Input: part model. Units: mm. Frame: model coordinates. A direction names the side the tool comes from. Coordinates: 2 decimals unless noted, no trailing zeros. Order: outer loops, then holes, each group sorted by start corner. A loop starts at its lowest first (then second) coordinate and runs counter-clockwise, first axis right, second up.
from build123d import *

# Parameters (mm, degrees)
BASE_DEPTH                  = 2
MUR_DEPTH                   = 15
ESQUISSE3_W                 = 4.5
ESQUISSE3_H                 = 4.5
FIXATION_VIS_DEPTH          = 13
CONG_1_R                    = 2
ESQUISSE4_R                 = 2.2
INSERT_M3_DEPTH             = 6
INSERT_M3_DIRECTION_2_REACH = 29.951
PASSE_CABLE_REACH           = 38.249
ESQUISSE5_R                 = 1
ESQUISSE8_W                 = 8
ESQUISSE8_H                 = 7.5
PATES_FIXATION_DEPTH        = 2
PASSAGE_VIS_REACH           = 34.33
ESQUISSE9_R                 = 1.6
CONG_10MM_R                 = 10
CONG_2MM_R                  = 2
CONG_1_5MM_R                = 1.5


with BuildPart() as part:
    # Esquisse1 → Base (new body)
    with BuildSketch(Plane(origin=(0, 0, 0), x_dir=(1, 0, 0), z_dir=(0, 1, 0))):
        with BuildLine():
            Line((-10.5, 20), (10.5, 20))
            ThreePointArc((10.5, 20), (11.914213562, 19.414213562), (12.5, 18))
            Line((12.5, 18), (12.5, -18))
            ThreePointArc((12.5, -18), (11.914213562, -19.414213562), (10.5, -20))
            Line((10.5, -20), (-10.5, -20))
            ThreePointArc((-10.5, -20), (-11.914213562, -19.414213562), (-12.5, -18))
            Line((-12.5, -18), (-12.5, 18))
            ThreePointArc((-12.5, 18), (-11.914213562, 19.414213562), (-10.5, 20))
        make_face()
    extrude(amount=BASE_DEPTH)

    # Esquisse2 → Mur (add)
    with BuildSketch(Plane(origin=(0, 2, 0), x_dir=(1, 0, 0), z_dir=(0, 1, 0))):
        with BuildLine():
            Line((-12.5, 18), (-12.5, -18))
            ThreePointArc((-12.5, -18), (-11.914213562, -19.414213562), (-10.5, -20))
            Line((-10.5, -20), (10.5, -20))
            ThreePointArc((10.5, -20), (11.914213562, -19.414213562), (12.5, -18))
            Line((12.5, -18), (12.5, 18))
            ThreePointArc((12.5, 18), (11.914213562, 19.414213562), (10.5, 20))
            Line((10.5, 20), (-10.5, 20))
            ThreePointArc((-10.5, 20), (-11.914213562, 19.414213562), (-12.5, 18))
        make_face()
        with BuildLine():
            ThreePointArc((-10.5, 18.5), (-10.853553391, 18.353553391), (-11, 18))
            Line((-11, 18), (-11, -18))
            ThreePointArc((-11, -18), (-10.853553391, -18.353553391), (-10.5, -18.5))
            Line((-10.5, -18.5), (10.5, -18.5))
            ThreePointArc((10.5, -18.5), (10.853553391, -18.353553391), (11, -18))
            Line((11, -18), (11, 18))
            ThreePointArc((11, 18), (10.853553391, 18.353553391), (10.5, 18.5))
            Line((10.5, 18.5), (-10.5, 18.5))
        make_face(mode=Mode.SUBTRACT)
    extrude(amount=MUR_DEPTH)

    # Esquisse3 → Fixation Vis (add)
    with BuildSketch(Plane(origin=(0, 2, 0), x_dir=(1, 0, 0), z_dir=(0, 1, 0))):
        with Locations((-8.75, 16.25)):
            Rectangle(ESQUISSE3_W, ESQUISSE3_H)
        with Locations((8.75, 16.25)):
            Rectangle(ESQUISSE3_W, ESQUISSE3_H)
        with Locations((8.75, -16.25)):
            Rectangle(ESQUISSE3_W, ESQUISSE3_H)
        with Locations((-8.75, -16.25)):
            Rectangle(ESQUISSE3_W, ESQUISSE3_H)
    extrude(amount=FIXATION_VIS_DEPTH)

    # Congé1
    cong_1_edges = [part.edges().sort_by_distance(p)[0] for p in [
        (6.5, 8.5, 14),
        (-6.5, 8.5, 14),
        (-6.5, 8.5, -14),
        (6.5, 8.5, -14),
    ]]
    fillet(cong_1_edges, radius=CONG_1_R)

    # Esquisse4 → Insert M3 (cut)
    with BuildSketch(Plane(origin=(0, 15, 0), x_dir=(1, 0, 0), z_dir=(0, 1, 0))):
        with Locations(Location((-9.5, 17, 0), (0, 0, 42.98588608))):
            Circle(ESQUISSE4_R)
        with Locations(Location((9.5, 17, 0), (0, 0, 90))):
            Circle(ESQUISSE4_R)
        with Locations(Location((9.5, -17, 0), (0, 0, 47.01411392))):
            Circle(ESQUISSE4_R)
        with Locations(Location((-9.5, -17, 0), (0, 0, 90))):
            Circle(ESQUISSE4_R)
    extrude(amount=-INSERT_M3_DEPTH, mode=Mode.SUBTRACT)

    # Esquisse4 → Insert M3 direction 2 (cut, up to next)
    with BuildSketch(Plane(origin=(0, 15, 0), x_dir=(1, 0, 0), z_dir=(0, 1, 0)), mode=Mode.PRIVATE) as insert_m3_direction_2_sk1:
        with Locations(Location((-9.5, 17, 0), (0, 0, 42.98588608))):
            Circle(ESQUISSE4_R)
    insert_m3_direction_2_tool1 = extrude(insert_m3_direction_2_sk1.sketch, amount=INSERT_M3_DIRECTION_2_REACH, mode=Mode.PRIVATE) & part.part
    # Esquisse4 → Insert M3 direction 2 (cut, up to next)
    with BuildSketch(Plane(origin=(0, 15, 0), x_dir=(1, 0, 0), z_dir=(0, 1, 0)), mode=Mode.PRIVATE) as insert_m3_direction_2_sk2:
        with Locations(Location((9.5, 17, 0), (0, 0, 90))):
            Circle(ESQUISSE4_R)
    insert_m3_direction_2_tool2 = extrude(insert_m3_direction_2_sk2.sketch, amount=INSERT_M3_DIRECTION_2_REACH, mode=Mode.PRIVATE) & part.part
    # Esquisse4 → Insert M3 direction 2 (cut, up to next)
    with BuildSketch(Plane(origin=(0, 15, 0), x_dir=(1, 0, 0), z_dir=(0, 1, 0)), mode=Mode.PRIVATE) as insert_m3_direction_2_sk3:
        with Locations(Location((9.5, -17, 0), (0, 0, 47.01411392))):
            Circle(ESQUISSE4_R)
    insert_m3_direction_2_tool3 = extrude(insert_m3_direction_2_sk3.sketch, amount=INSERT_M3_DIRECTION_2_REACH, mode=Mode.PRIVATE) & part.part
    # Esquisse4 → Insert M3 direction 2 (cut, up to next)
    with BuildSketch(Plane(origin=(0, 15, 0), x_dir=(1, 0, 0), z_dir=(0, 1, 0)), mode=Mode.PRIVATE) as insert_m3_direction_2_sk4:
        with Locations(Location((-9.5, -17, 0), (0, 0, 90))):
            Circle(ESQUISSE4_R)
    insert_m3_direction_2_tool4 = extrude(insert_m3_direction_2_sk4.sketch, amount=INSERT_M3_DIRECTION_2_REACH, mode=Mode.PRIVATE) & part.part
    add(insert_m3_direction_2_tool1.solids().sort_by_distance((-9.5, 15, -17))[0], mode=Mode.SUBTRACT)
    add(insert_m3_direction_2_tool2.solids().sort_by_distance((9.5, 15, -17))[0], mode=Mode.SUBTRACT)
    add(insert_m3_direction_2_tool3.solids().sort_by_distance((9.5, 15, 17))[0], mode=Mode.SUBTRACT)
    add(insert_m3_direction_2_tool4.solids().sort_by_distance((-9.5, 15, 17))[0], mode=Mode.SUBTRACT)

    # Esquisse5 → Passe-Cable (cut, up to next)
    with BuildSketch(Plane.ZY.offset(12.5), mode=Mode.PRIVATE) as passe_cable_sk1:
        with Locations((-10, 6)):
            Circle(ESQUISSE5_R)
    passe_cable_tool1 = extrude(passe_cable_sk1.sketch, amount=-PASSE_CABLE_REACH, mode=Mode.PRIVATE) & part.part
    add(passe_cable_tool1.solids().sort_by_distance((-12.5, 6, -10))[0], mode=Mode.SUBTRACT)

    # Esquisse8 → Pates fixation (add)
    with BuildSketch(Plane(origin=(0, 0, 0), x_dir=(1, 0, 0), z_dir=(0, 1, 0))):
        with Locations((16.5, 0)):
            Rectangle(ESQUISSE8_W, ESQUISSE8_H)
        with Locations((-16.5, 0)):
            Rectangle(ESQUISSE8_W, ESQUISSE8_H)
    extrude(amount=PATES_FIXATION_DEPTH)

    # Esquisse9 → Passage_Vis (cut, up to next)
    with BuildSketch(Plane(origin=(0, 2, 0), x_dir=(1, 0, 0), z_dir=(0, 1, 0)), mode=Mode.PRIVATE) as passage_vis_sk1:
        with Locations(Location((-17.5, 0, 0), (0, 0, 270))):
            Circle(ESQUISSE9_R)
    passage_vis_tool1 = extrude(passage_vis_sk1.sketch, amount=-PASSAGE_VIS_REACH, mode=Mode.PRIVATE) & part.part
    # Esquisse9 → Passage_Vis (cut, up to next)
    with BuildSketch(Plane(origin=(0, 2, 0), x_dir=(1, 0, 0), z_dir=(0, 1, 0)), mode=Mode.PRIVATE) as passage_vis_sk2:
        with Locations(Location((17.5, 0, 0), (0, 0, 270))):
            Circle(ESQUISSE9_R)
    passage_vis_tool2 = extrude(passage_vis_sk2.sketch, amount=-PASSAGE_VIS_REACH, mode=Mode.PRIVATE) & part.part
    add(passage_vis_tool1.solids().sort_by_distance((-17.5, 2, 0))[0], mode=Mode.SUBTRACT)
    add(passage_vis_tool2.solids().sort_by_distance((17.5, 2, 0))[0], mode=Mode.SUBTRACT)

    # Congé_10mm
    # the kernel refuses this fillet: 10 mm, written as the material it adds along each edge
    with BuildSketch(Plane(origin=(12.5, 0, 3.75), x_dir=(0, 0, 1), z_dir=(0, 1, 0)), Plane(origin=(-12.5, 0, -3.75), x_dir=(0, 0, -1), z_dir=(0, 1, 0))) as cong_10mm_piece_1:
        with BuildLine():
            CenterArc((9.797958971, 10), CONG_10MM_R, 191.536959033, 78.463040967)
            Line((0, 8), (-0.195959179, 7.96))
            ThreePointArc((-0.195959179, 7.96), (-0.2, 4), (-0.2, 0))
            Line((-0.2, 0), (0, -0.2))
            Line((0, -0.2), (9.797958971, -0.2))
            Line((9.797958971, -0.2), (9.797958971, 0))
        make_face()
    extrude(amount=2)
    with BuildSketch(Plane(origin=(12.5, 0, -3.75), x_dir=(0, 0, -1), z_dir=(0, 1, 0)), Plane(origin=(-12.5, 0, 3.75), x_dir=(0, 0, 1), z_dir=(0, 1, 0))) as cong_10mm_piece_2:
        with BuildLine():
            CenterArc((9.797958971, -10), CONG_10MM_R, 90, 78.463040967)
            Line((0, -8), (-0.195959179, -7.96))
            ThreePointArc((-0.195959179, -7.96), (-0.2, -4), (-0.2, 0))
            Line((-0.2, 0), (0, 0.2))
            Line((0, 0.2), (9.797958971, 0.2))
            Line((9.797958971, 0.2), (9.797958971, 0))
        make_face()
    extrude(amount=2)

    # Congé_2mm
    # the kernel refuses this fillet: 2 mm, written as the material it takes off along each edge
    with BuildSketch(Plane(origin=(20.5, -3.78937382, 3.75), x_dir=(-0.9636113749942804, 0, 0.26730716036356444), z_dir=(0, 1, 0)), Plane(origin=(-20.5, -3.78937382, -3.75), x_dir=(0.9636113749942804, 0, -0.26730716036356456), z_dir=(0, 1, 0))) as cong_2mm_piece_1:
        with BuildLine():
            CenterArc((1.522052048, -1.995207807), CONG_2MM_R, 93.967130801, 70.528779366)
            Line((-0.405170702, -1.460593487), (0, 0))
            ThreePointArc((0, 0), (0.69184184, -0.023960963), (1.38368368, 0))
        make_face()
    extrude(amount=9.578747639, mode=Mode.SUBTRACT)
    with BuildSketch(Plane(origin=(20.5, -3.78937382, -3.75), x_dir=(-0.9636113749942801, 0, -0.2673071603635657), z_dir=(0, 1, 0))) as cong_2mm_piece_2:
        with BuildLine():
            CenterArc((1.522052048, 1.995207807), CONG_2MM_R, 195.504089834, 70.528779366)
            Line((-0.405170702, 1.460593487), (0, 0))
            ThreePointArc((0, 0), (0.69184184, 0.023960963), (1.38368368, 0))
        make_face()
    extrude(amount=9.578747639, mode=Mode.SUBTRACT)
    with BuildSketch(Plane(origin=(-20.5, -3.78937382, 3.75), x_dir=(0, 0, -1), z_dir=(0, 1, 0))) as cong_2mm_piece_3:
        with BuildLine():
            CenterArc((1.515749528, -2), CONG_2MM_R, 90, 70.528779366)
            ThreePointArc((-0.369868555, -1.333333333), (-0.161845221, -0.673071604), (0, 0))
            Line((0, 0), (1.515749528, 0))
        make_face()
    extrude(amount=9.578747639, mode=Mode.SUBTRACT)

    # Congé_1,5mm
    cong_1_5mm_edges = [part.edges().sort_by_distance(p)[0] for p in [
        (12.5, 2, 0),
        (-12.5, 2, 0),
    ]]
    fillet(cong_1_5mm_edges, radius=CONG_1_5MM_R)


solid = part.part
Item 1: Pin query (flat end, axial travel): pin 1 Ø1.5 at (y, z) = (5, -7) entering from +X; pin 2 Ø6.5 at (x, z) = (0, -2.5) entering from +Y; pin 3 Ø2 at (x, z) = (10.5, -17) entering from +Y. Return the tip coordinate at first contact, or that it passes through.
Response values:
pin 1: stops at x = 12.5
pin 2: stops at y = 2
pin 3: stops at y = 9
Item 2: Ray query, probe 1 along Z at (x, y) = (9.5, 13.2); probe 2 along X at (y, z) = (12.8, 17); probe 3 along X at (y, z) = (14.25, 6). Return the intervals inside material, ascending.
Response values:
probe 1: z = -20 to -19.2, -14.8 to -14, 14 to 14.8, 19.2 to 20
probe 2: x = -12.5 to -11.7, -7.3 to -6.5, 6.5 to 7.3, 11.7 to 12.5
probe 3: x = -12.5 to -11, 11 to 12.5
Item 3: Cut plane A-A on y = 10. Return loops of the section in (x, z).
Response values:
outline: (-12.5, -18) arc R2 ccw to (-10.5, -20) - (10.5, -20) arc R2 ccw to (12.5, -18) - (12.5, 18) arc R2 ccw to (10.5, 20) - (-10.5, 20) arc R2 ccw to (-12.5, 18) - close; hole circle Ø4.4 at (-9.5, -17); hole circle Ø4.4 at (-9.5, 17); hole (-11, -14) - (-8.5, -14) arc R2 cw to (-6.5, -16) - (-6.5, -18.5) - (6.5, -18.5) - (6.5, -16) arc R2 cw to (8.5, -14) - (11, -14) - (11, 14) - (8.5, 14) arc R2 cw to (6.5, 16) - (6.5, 18.5) - (-6.5, 18.5) - (-6.5, 16) arc R2 cw to (-8.5, 14) - (-11, 14) - close; hole circle Ø4.4 at (9.5, -17); hole circle Ø4.4 at (9.5, 17)
Item 4: Cut plane B-B on z = 0. Return loops of the section in (x, y), then the cut area to 3 significant figures.
Response values:
outline: (-20.5, 0) - (-19.1, 0) - (-19.1, 2) - (-20.5, 2) - close; (-15.9, 0) - (15.9, 0) - (15.9, 2) - (14, 2) arc R1.5 cw to (12.5, 3.5) - (12.5, 17) - (11, 17) - (11, 2) - (-11, 2) - (-11, 17) - (-12.5, 17) - (-12.5, 3.5) arc R1.5 cw to (-14, 2) - (-15.9, 2) - close; (19.1, 0) - (20.5, 0) - (20.5, 2) - (19.1, 2) - close
area: 115 mm2
Item 5: Access query for faces 5 (the face through (-10, 9, 17)), 6 (the face through (15, 2, 0)), 7 (the face through (-11.93, 8.38, 19.4)). Directions: +Z, -Z, +X, -X, +Y, -Y. A direction counts if a zero-diameter tool reaches every point of the face in a straight line with its end or side. Return the directions, or none.
Response values:
face 5: +Y
face 6: +Z, -Z, +X, +Y
face 7: +Z, -X, +Y, -Y
Item 6: Draft query along X for faces 1 (the face through (9, 9, -17)), 2 (the face through (11.9, 8.38, 19.43)), 3 (the face through (-20.123, 0.986, -3.403)), 4 (the face through (-10, 8, -14)). Return one class per face: pulls with the +X half, pulls with the -X half, needs draft (parallel to the pull), parting line crosses it, or undercut.
Response values:
face 1: undercut
face 2: pulls with the +X half
face 3: pulls with the -X half
face 4: undercut
Item 7: Cut plane C-C on y = 1.5. Return loops of the section in (x, z).
Response values:
outline: (-20.5, -2.23) arc R2 ccw to (-19.17, -4.12) arc R10 cw to (-12.5, -13.55) - (-12.5, -18) arc R2 ccw to (-10.5, -20) - (10.5, -20) arc R2 ccw to (12.5, -18) - (12.5, -13.55) arc R10 cw to (19.17, -4.12) arc R2 ccw to (20.5, -2.23) - (20.5, 2.23) arc R2 ccw to (19.17, 4.12) arc R10 cw to (12.5, 13.55) - (12.5, 18) arc R2 ccw to (10.5, 20) - (-10.5, 20) arc R2 ccw to (-12.5, 18) - (-12.5, 13.55) arc R10 cw to (-19.17, 4.12) arc R2 ccw to (-20.5, 2.23) - close; hole circle Ø3.2 at (-17.5, 0); hole circle Ø3.2 at (17.5, 0)
Item 8: Cut plane D-D on x = -17.5. Return loops of the section in (y, z), then the cut area to 3 significant figures.
Response values:
outline: (0, -4.89) - (2, -4.89) - (2, -1.6) - (0, -1.6) - close; (0, 1.6) - (2, 1.6) - (2, 4.89) - (0, 4.89) - close
area: 13.2 mm2
